from build123d import *

# Parameters (mm, degrees)
F0_W     = 7.62
F0_H     = 38.1
F0_W_2   = 12.7
F1_DEPTH = 127
F2_W     = 87.2650571496
F2_H     = 7.4778180569
F3_DEPTH = 38.1
F5_W     = 2.54
F5_H     = 6.1494747632
F6_DEPTH = 5.08


with BuildPart() as f1:
    # F0 (on Front) → F1 (new body)
    with BuildSketch(Plane.XZ):
        Polygon((-64.6448548068, -3.3340927702), (-64.6448548068, -20.8513359327), (42.9402023428, -20.8513359327), (42.9402023428, -3.3340927702), (30.2402023428, -3.3340927702), (-57.0248548068, -3.3340927702), align=None)
        with Locations((-60.8348548068, 15.7159072298)):
            Rectangle(F0_W, F0_H)
        with Locations((36.5902023428, 15.7159072298)):
            Rectangle(F0_W_2, F0_H)
    extrude(amount=F1_DEPTH)

    # F2 (on face) → F3 (join)
    with BuildSketch(Plane.XY.offset(-3.3340927702)):
        with Locations((-13.392326232, -3.7389090285)):
            Rectangle(F2_W, F2_H)
    extrude(amount=F3_DEPTH)

    # F5 (on face) → F6 (join)
    with BuildSketch(Plane.XZ.offset(127)):
        Polygon((30.2402023428, -3.3340927702), (30.2402023428, 33.2476731723), (17.5402023428, 33.2476731723), (17.5402023428, 22.0181959489), (17.5402023428, -3.3340927702), align=None)
        Polygon((17.5402023428, -3.3340927702), (17.5402023428, 22.0181959489), (7.3802023428, 22.0181959489), (7.3802023428, 15.3339850341), (7.3802023428, -3.3340927702), align=None)
        Polygon((-0.2397976572, -3.3340927702), (7.3802023428, -3.3340927702), (7.3802023428, 15.3339850341), (-0.2397976572, 15.3339850341), (-0.2397976572, 8.1150363277), align=None)
        Polygon((-5.3197976572, -3.3340927702), (-0.2397976572, -3.3340927702), (-0.2397976572, 8.1150363277), (-5.3197976572, 8.1150363277), (-5.3197976572, 2.8153819931), align=None)
        with Locations((-6.5897976572, -0.2593553885)):
            Rectangle(F5_W, F5_H)
    extrude(amount=-F6_DEPTH)


solid = f1.part
Work out the finished part from the listing and answer in its coordinate system (mm). A direction names the side the tool comes from. Round coordinates to 2 decimals unless told otherwise and drop trailing zeros. Write each loop counter-clockwise with the first axis right and the second up, starting at its lowest first coordinate (ties: lowest second). Pieces come first, ordered by that corner, then holes. Notation, with made-up numbers: M 18,68.25 L 61,68.25 A26 ccw 61,106.25 Z; hole C 22,25.5 d8. An arc over 180 degrees is marked long. Use a Markdown table: item, result.
1) Determine the mould class of faces 1 (the face through (-13, -66, -3.334)), 2 (the face through (-12, 0, 7)), 3 (the face through (42.94, -63, 7)) for opening direction X: pulls with the +X half, pulls with the -X half, needs draft (parallel to the pull), parting line crosses it, or undercut.
Taken from the geometry:
| item | result |
|---|---|
| face 1 | undercut |
| face 2 | needs draft |
| face 3 | pulls with the +X half |
2) The part is cut by section D-D on z = 10. Give the vertices of the cut face in (x, y), plus the area to 3 significant figures.
Taken from the geometry:
| item | result |
|---|---|
| outline | M -64.64,-127 L -57.02,-127 L -57.02,-7.48 L 30.24,-7.48 L 30.24,-121.92 L -0.24,-121.92 L -0.24,-127 L 42.94,-127 L 42.94,0 L -64.64,0 Z |
| area | 3,390 mm2 |
3) Flat-ended cylindrical pins translate along their axes: pin 1 (1.5 mm diameter, centred on x = -2, y = -123.5, fed in from +Z); pin 2 (2.5 mm diameter, centred on x = 4, y = -125, fed in from +Z); pin 3 (3 mm diameter, centred on x = -42.5, y = -113.5, fed in from +Z). Find the tip coordinate at first contact, or state that the pin passes through.
Taken from the geometry:
| item | result |
|---|---|
| pin 1 | stops at z = 8.12 |
| pin 2 | stops at z = 15.33 |
| pin 3 | stops at z = -3.33 |
4) The part is cut by section C-C on y = -50.5. Give the vertices of the cut face in (x, z), plus the area to 3 significant figures.
Taken from the geometry:
| item | result |
|---|---|
| outline | M -64.64,-20.85 L 42.94,-20.85 L 42.94,34.77 L 30.24,34.77 L 30.24,-3.33 L -57.02,-3.33 L -57.02,34.77 L -64.64,34.77 Z |
| area | 2,660 mm2 |
5) The part is cut by section B-B on z = 18. Give the vertices of the cut face in (x, y).
Taken from the geometry:
| item | result |
|---|---|
| outline | M -64.64,-127 L -57.02,-127 L -57.02,-7.48 L 30.24,-7.48 L 30.24,-121.92 L 7.38,-121.92 L 7.38,-127 L 42.94,-127 L 42.94,0 L -64.64,0 Z |
6) Consider line 1 (X direction, y = -86, z = 31); line 2 (Z direction, x = -13, y = -89.5); line 3 (Y direction, x = -3.5, z = 28). Determine where each line is inside the solid, lowest interval first. Write a range as [from, to].
Taken from the geometry:
| item | result |
|---|---|
| line 1 | x = [-64.64, -57.02], [30.24, 42.94] |
| line 2 | z = [-20.85, -3.33] |
| line 3 | y = [-7.48, 0] |
7) The part is cut by section A-A on x = 11.5. Give the vertices of the cut face in (y, z), plus the area to 3 significant figures.
Taken from the geometry:
| item | result |
|---|---|
| outline | M -127,-20.85 L 0,-20.85 L 0,34.77 L -7.48,34.77 L -7.48,-3.33 L -121.92,-3.33 L -121.92,22.02 L -127,22.02 Z |
| area | 2,640 mm2 |
8) Which of the six approach directions +Z, -Z, +X, -X, +Y, -Y give full straight-line access (tool end or side, diameter ignored) to faces 4 (the face through (0, -127, 1)), 5 (the face through (7.38, -124, 19)), 6 (the face through (15, -121.92, 11))?
Taken from the geometry:
| item | result |
|---|---|
| face 4 | +Z, -Z, +X, -X, -Y |
| face 5 | +Z, -Y |
| face 6 | +Z |
